Geometry: final body of the model. Coordinates: model frame, mm. Face numbers are marked on the shaded views. Give positions to 0.01 mm unless a question says otherwise; leave off trailing zeros. Write each loop counter-clockwise with the first axis right and the second up, starting at its lowest first coordinate (ties: lowest second). Pieces come first, ordered by that corner, then holes.
from build123d import *

# Parameters (mm, degrees)
BOSS_EXTRUDE2_DEPTH = 2.54
SKETCH1_5_R         = 4.233333332
BOSS_EXTRUDE3_DEPTH = 7.62
SKETCH1_6_R         = 6.096
CUT_EXTRUDE1_DEPTH  = 3.5400001
SKETCH4_R           = 8.763
CUT_EXTRUDE2_DEPTH  = 0.508


with BuildPart() as part:
    # Sketch1 → Boss-Extrude2 (new body)
    with BuildSketch(Plane.XY):
        with BuildLine():
            ThreePointArc((-126.772670279, 46.57403283), (-115.299991188, 26.89475243), (-126.772670279, 7.21547203))
            add(Edge.make_bspline(
                [(-172.474815081, 26.89475243), (-172.473819891, 26.558530991), (-172.419747256, 25.722281586), (-172.09778315, 24.251653169), (-171.305841422, 22.419535029), (-169.889362805, 20.390404018), (-167.799877065, 18.323101104), (-165.058549527, 16.327195732), (-161.711634875, 14.468005136), (-157.809164116, 12.783310723), (-153.398533522, 11.295434272), (-148.523738698, 10.01761911), (-143.225981341, 8.957316813), (-137.544438784, 8.118011859), (-132.01714462, 7.550633923), (-128.386674126, 7.303527814), (-126.772670279, 7.21547203)],
                knots=[0.5, 0.5, 0.5, 0.5, 0.502166769, 0.505390167, 0.509655974, 0.514947682, 0.521244711, 0.528520886, 0.536744945, 0.54588136, 0.555890751, 0.566730119, 0.57835299, 0.590709588, 0.603747039, 0.614168613, 0.614168613, 0.614168613, 0.614168613], degree=3))
            add(Edge.make_bspline(
                [(-172.474815081, 26.89475243), (-172.473819891, 27.230973869), (-172.419747256, 28.067223274), (-172.09778315, 29.537851691), (-171.305841422, 31.369969831), (-169.889362805, 33.399100842), (-167.799877065, 35.466403756), (-165.058549528, 37.462309128), (-161.711634876, 39.321499724), (-157.809164116, 41.006194136), (-153.398533523, 42.494070588), (-148.523738699, 43.77188575), (-143.225981342, 44.832188047), (-137.544438785, 45.671493001), (-132.01714462, 46.238870937), (-128.386674126, 46.485977046), (-126.772670279, 46.57403283)],
                knots=[0.5, 0.5, 0.5, 0.5, 0.502166769, 0.505390167, 0.509655974, 0.514947682, 0.521244711, 0.528520886, 0.536744945, 0.54588136, 0.555890751, 0.566730119, 0.57835299, 0.590709588, 0.603747039, 0.614168613, 0.614168613, 0.614168613, 0.614168613], degree=3))
        make_face()
    extrude(amount=BOSS_EXTRUDE2_DEPTH)

    # Sketch1_5 → Boss-Extrude3 (add)
    with BuildSketch(Plane.XY):
        with Locations((-159.081098581, 26.89475243)):
            Circle(SKETCH1_5_R)
    extrude(amount=-BOSS_EXTRUDE3_DEPTH)

    # Sketch1_6 → Cut-Extrude1 (cut, through all)
    with BuildSketch(Plane.XY):
        with Locations((-137.914431916, 26.89475243)):
            Circle(SKETCH1_6_R)
    extrude(amount=CUT_EXTRUDE1_DEPTH, mode=Mode.SUBTRACT)

    # Sketch4 → Cut-Extrude2 (cut)
    with BuildSketch(Plane.XY.offset(2.54)):
        with Locations((-137.914431916, 26.89475243)):
            Circle(SKETCH4_R)
    extrude(amount=-CUT_EXTRUDE2_DEPTH, mode=Mode.SUBTRACT)


solid = part.part
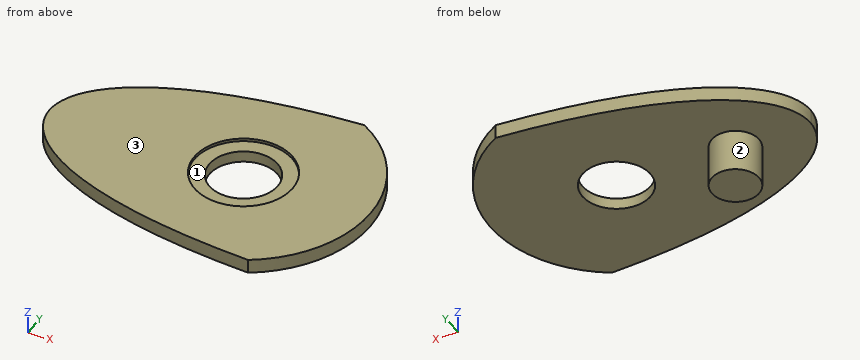
Q1. Pin query (flat end, axial travel): P1, Ø19.5, axis at x = -137.91, y = 26.89, coming from the -Z side; P2, Ø6, axis at x = -144, z = -1.5, coming from the +Y side; P3, Ø14, axis at x = -138, y = 27, coming from the +Z side. Return the tip coordinate at first contact, or that it passes through.
Filled sheet:
P1: stops at z = 0
P2: stops at y = 45.09
P3: stops at z = 2.03
Q2. Section B-B on x = -125. Output: boundary loops of the cut face in (y, z).
Filled sheet:
outline: (8.33, 0) - (45.46, 0) - (45.46, 2.54) - (8.33, 2.54) - close
Q3. Section A-A on z = -5.75. Output: boundary loops of the cut face in (x, y), plus the area to 3 significant figures.
Filled sheet:
outline: circle Ø8.47 at (-159.08, 26.89)
area: 56.3 mm2
Q4. Ray query, line 1 along Z through (x, y) = (-119.5, 16); line 2 along X through (y, z) = (22.5, 2); line 3 along X through (y, z) = (28, -5.75). Return the intervals inside material, ascending.
Filled sheet:
line 1: z = 0 to 2.54
line 2: x = -171.26 to -142.14, -133.69 to -115.73
line 3: x = -163.17 to -154.99
Q5. Pull-direction query (Y, two-part tool) for the marked faces 1, 2 and 3; classes: released by +Y, released by -Y, zero draft, split by the parting line, or undercut.
Filled sheet:
face 1: undercut
face 2: split by the parting line
face 3: zero draft
